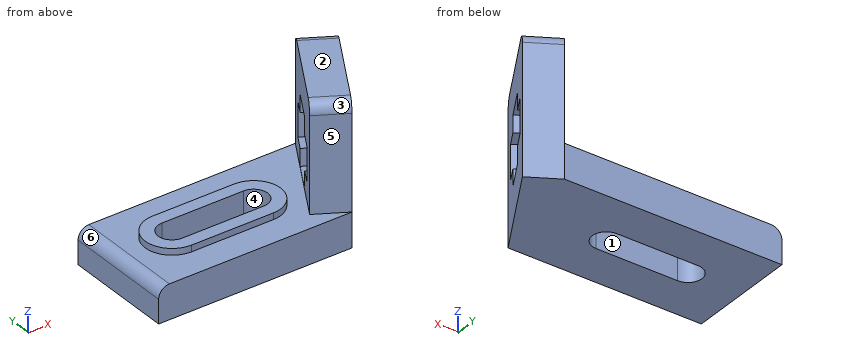
```python
from build123d import *

# Parameters (mm, degrees)
F1_DEPTH  = 32.5
F5_DEPTH  = 16
F6_R      = 5
F8_DEPTH  = 3
F9_DEPTH  = 16.001
F11_DEPTH = 20
F12_R     = 5


with BuildPart() as f1:
    # F0 (on Top) → F1 (new body, symmetric)
    with BuildSketch(Plane.XY):
        Polygon((-13.8564064606, 8), (0, 0), (25, 43.3012701892), (11.1435935394, 51.3012701892), align=None)
    extrude(amount=F1_DEPTH, both=True)

    # F4 (on face) → F5 (join)
    with BuildSketch(Plane(origin=(0, 0, -32.5), x_dir=(1, 0, 0), z_dir=(0, 0, -1))):
        Polygon((-13.8564064606, -8), (0, 0), (-90, 0), (-90, -51.3012701892), (11.1435935394, -51.3012701892), align=None)
    extrude(amount=-F5_DEPTH)

    # F6
    f6_edges = [f1.edges().sort_by_distance(p)[0] for p in [
        (-6.928203, 4, 32.5),
        (18.071797, 47.30127, 32.5),
    ]]
    fillet(f6_edges, radius=F6_R)

    # F7 (on face) → F8 (join)
    with BuildSketch(Plane.XY.offset(-16.5)):
        with BuildLine():
            ThreePointArc((-65, 38.1506350946), (-77.5, 25.6506350946), (-65, 13.1506350946))
            Line((-65, 13.1506350946), (-65, 19.1506350946))
            ThreePointArc((-65, 19.1506350946), (-71.5, 25.6506350946), (-65, 32.1506350946))
            Line((-65, 32.1506350946), (-65, 38.1506350946))
        make_face()
        with BuildLine():
            Line((-65, 19.1506350946), (-65, 13.1506350946))
            ThreePointArc((-65, 13.1506350946), (-58.876275643, 14.7533877358), (-54.322921748, 19.1506350946))
            Line((-54.322921748, 19.1506350946), (-65, 19.1506350946))
        make_face()
        with BuildLine():
            Line((-65, 13.1506350946), (-27, 13.1506350946))
            ThreePointArc((-27, 13.1506350946), (-33.123724357, 14.7533877358), (-37.677078252, 19.1506350946))
            Line((-37.677078252, 19.1506350946), (-54.322921748, 19.1506350946))
            ThreePointArc((-54.322921748, 19.1506350946), (-58.876275643, 14.7533877358), (-65, 13.1506350946))
        make_face()
        with BuildLine():
            Line((-27, 19.1506350946), (-27, 13.1506350946))
            ThreePointArc((-27, 13.1506350946), (-18.1611652352, 16.8118003298), (-14.5, 25.6506350946))
            ThreePointArc((-14.5, 25.6506350946), (-18.1611652352, 34.4894698594), (-27, 38.1506350946))
            Line((-27, 38.1506350946), (-27, 32.1506350946))
            ThreePointArc((-27, 32.1506350946), (-22.4038059223, 30.2468291723), (-20.5, 25.6506350946))
            ThreePointArc((-20.5, 25.6506350946), (-22.4038059223, 21.0544410169), (-27, 19.1506350946))
        make_face()
        with BuildLine():
            ThreePointArc((-37.677078252, 19.1506350946), (-33.123724357, 14.7533877358), (-27, 13.1506350946))
            Line((-27, 13.1506350946), (-27, 19.1506350946))
            Line((-27, 19.1506350946), (-37.677078252, 19.1506350946))
        make_face()
        with BuildLine():
            Line((-37.677078252, 32.1506350946), (-27, 32.1506350946))
            Line((-27, 32.1506350946), (-27, 38.1506350946))
            ThreePointArc((-27, 38.1506350946), (-33.123724357, 36.5478824535), (-37.677078252, 32.1506350946))
        make_face()
        with BuildLine():
            ThreePointArc((-54.322921748, 32.1506350946), (-58.876275643, 36.5478824535), (-65, 38.1506350946))
            Line((-65, 38.1506350946), (-65, 32.1506350946))
            Line((-65, 32.1506350946), (-54.322921748, 32.1506350946))
        make_face()
        with BuildLine():
            Line((-27, 38.1506350946), (-65, 38.1506350946))
            ThreePointArc((-65, 38.1506350946), (-58.876275643, 36.5478824535), (-54.322921748, 32.1506350946))
            Line((-54.322921748, 32.1506350946), (-37.677078252, 32.1506350946))
            ThreePointArc((-37.677078252, 32.1506350946), (-33.123724357, 36.5478824535), (-27, 38.1506350946))
        make_face()
    extrude(amount=F8_DEPTH)

    # F9 (cut, through all): a face of the model
    f9_faces = [f1.faces().sort_by_distance(p)[0] for p in [
        (-46, 25.6506350946, -16.5),
    ]]
    extrude(f9_faces, amount=-F9_DEPTH, mode=Mode.SUBTRACT)

    # F10 (on face) → F11 (cut)
    with BuildSketch(Plane(origin=(0, 0, 0), x_dir=(0.5, 0.8660254038, 0), z_dir=(0.8660254038, -0.5, 0))):
        Polygon((33, -8), (41, -8), (41, 8), (33, 8), (33, 16), (17, 16), (17, 8), (9, 8), (9, -8), (17, -8), (17, -16), (33, -16), align=None)
    extrude(amount=-F11_DEPTH, mode=Mode.SUBTRACT)

    # F12
    f12_edges = [f1.edges().sort_by_distance(p)[0] for p in [
        (-90, 25.650635, -16.5),
    ]]
    fillet(f12_edges, radius=F12_R)


solid = f1.part
```
Verification items for the finished model (mm, model axes). Face numbers are marked on the shaded views. A direction names the side the tool comes from. Coordinates: 2 decimals unless noted, no trailing zeros. Write each loop counter-clockwise with the first axis right and the second up, starting at its lowest first coordinate (ties: lowest second). Pieces come first, ordered by that corner, then holes. Notation, with made-up numbers: M -22,-13 L 10,-13 A5 cw 10,-6 Z; hole C -20.75,-18 d3. An arc over 180 degrees is marked long. Answer as a JSON object with one key per item and string values. Group by question number.
(1) Release check for a two-part mould opening along Y. For the marked faces 1, 2 and 3 record: +Y half, -Y half, draft (parallel to the pull), parting line (faces both ways), or undercut.
(2) Cross-section at C-C, the plane z = -24. Record the cut outline in (x, y), and give its area (3 significant figures).
(3) Tool access check on the marked faces 4, 5 and 6. Record the directions out of +Z, -Z, +X, -X, +Y, -Y that give a thin tool (end or side, any length) a straight path to the whole face; none if there is none.
(4) Cross-section at D-D, the plane x = -16. Record the cut outline in (y, z), and give its area (3 significant figures).
(5) Material ranges on line 1 (Y direction, x = -65, z = -14); line 2 (Z direction, x = -36, y = 8); line 3 (X direction, y = 24, z = -14.5), recorded low to high.
(6) Cross-section at A-A, the plane z = 13. Record the cut outline in (x, y).
(7) Gauge pin test, flat ends, axial feed: pin 1 (5.5 mm diameter, centred on x = -46, z = -22.5, fed in from -Y); pin 2 (2.5 mm diameter, centred on x = -51, z = -14.5, fed in from +Y); pin 3 (4 mm diameter, centred on y = 46, z = -22.5, fed in from +X); pin 4 (1.5 mm diameter, centred on x = -14.5, y = 44.5, fed in from +Z). Record the tip position at first contact, or that the pin passes through.
(8) Cross-section at B-B, the plane y = 17. Record the cut outline in (x, z), and give its area (3 significant figures).
Reply:
{
 "1": {"face 1": "undercut", "face 2": "draft", "face 3": "-Y half"},
 "2": {"outline": "M -90,0 L 0,0 L 25,43.3 L 11.14,51.3 L -90,51.3 Z; hole M -65,19.15 L -27,19.15 A6.5 ccw -27,32.15 L -65,32.15 A6.5 ccw Z", "area": "4,680 mm²"},
 "3": {"face 4": "+Z, -Z", "face 5": "+Z, -X, -Y", "face 6": "+Z, -X, +Y, -Y"},
 "4": {"outline": "M 0,-32.5 L 51.3,-32.5 L 51.3,-16.5 L 31.59,-16.5 L 31.59,-13.5 L 19.71,-13.5 L 19.71,-16.5 L 0,-16.5 Z", "area": "856 mm²"},
 "5": {"line 1": "13.15 to 19.15, 32.15 to 38.15", "line 2": "-32.5 to -16.5", "line 3": "-77.39 to -71.29, -20.71 to -14.61"},
 "6": {"outline": "M -13.86,8 L 0,0 L 8.5,14.72 L -5.36,22.72 Z; M 2.64,36.58 L 16.5,28.58 L 25,43.3 L 11.14,51.3 Z"},
 "7": {"pin 1": "y = 0", "pin 2": "y = 38.15", "pin 3": "x = 23.79", "pin 4": "z = -16.5"},
 "8": {"outline": "M -90,-32.5 L 9.81,-32.5 L 9.81,-16 L 4.56,-16 L 4.56,-8 L -8.66,-8 L -8.66,-16.5 L -17.98,-16.5 L -17.98,-13.5 L -74.02,-13.5 L -74.02,-16.5 L -85,-16.5 A5 ccw -90,-21.5 Z; M -8.66,8 L 4.56,8 L 4.56,16 L 9.81,16 L 9.81,32.5 L -8.66,32.5 Z", "area": "2,290 mm²"}
}
